Geometry check sheet. Reference: drawing and pictorial views, mm from the part's lowest x, y, z. Give positions to 0.01 mm unless a question says otherwise; leave off trailing zeros. Order: outer loops, then holes, each group sorted by start corner. A loop starts at its lowest first (then second) coordinate and runs counter-clockwise, first axis right, second up. Notation, with made-up numbers: (13, -25.75) -> (20, -25.75) arc R26 cw to (20, -7.75) -> close; hole circle Ø9 at (45, -3.5). An arc over 180 degrees is marked (long way). Write each question's results on one line, items separated by ' | '. Start each with the question number.
1. Cross-section at A-A, the plane x = 59. Enter the section's corners in (y, z).
2. Depth check by flat-ended pin: pin 1 Ø1 at (x, z) = (38.5, 1) entering from -Y. Enter the tip coordinate at first touch or a pass-through.
3. Cross-section at C-C, the plane y = 73. Enter the section's corners in (x, z), then the cut area to 3 significant figures.
4. Cross-section at D-D, the plane z = 0.55. State how many separate pieces and enclosed holes the cut face has, then the cut area to 3 significant figures.
5. Cross-section at B-B, the plane x = 12. Enter the section's corners in (y, z).
6. Material ranges on L1, parallel to Y at x = 12, z = 1.1; L2, parallel to Y at x = 43, z = 0.95; L3, parallel to Y at x = 59, z = 1.3, recorded low to high. Write a range as from..to.
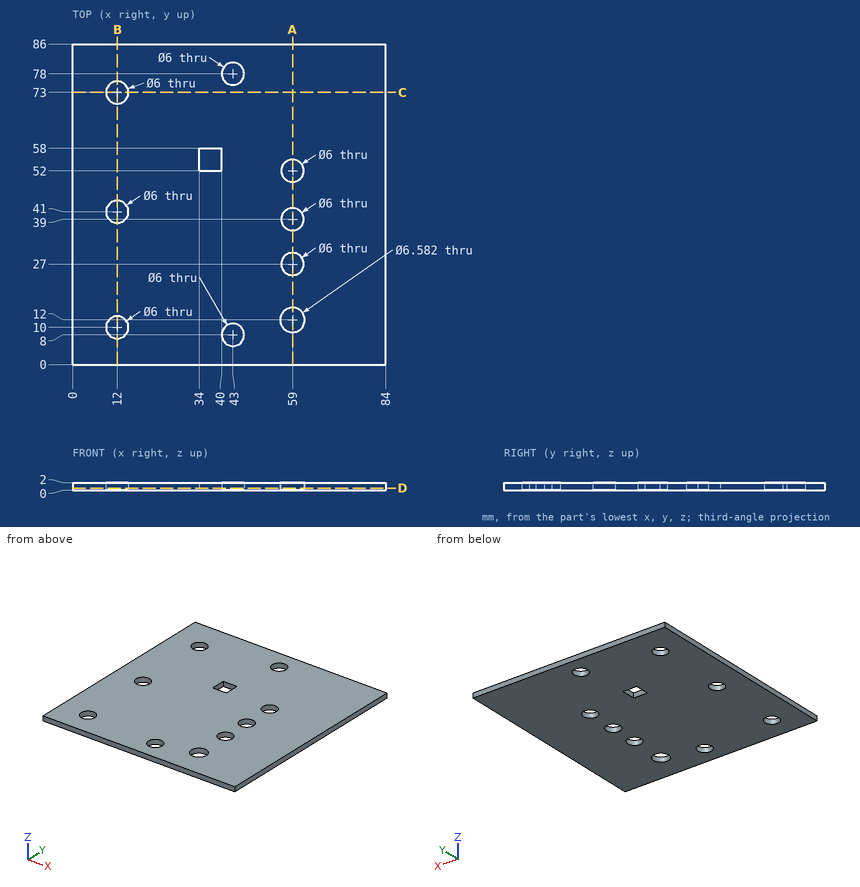
Results below:
1) outline: (0, 0) -> (8.71, 0) -> (8.71, 2) -> (0, 2) -> close; (15.29, 0) -> (24, 0) -> (24, 2) -> (15.29, 2) -> close; (30, 0) -> (36, 0) -> (36, 2) -> (30, 2) -> close; (42, 0) -> (49, 0) -> (49, 2) -> (42, 2) -> close; (55, 0) -> (86, 0) -> (86, 2) -> (55, 2) -> close
2) pin 1: stops at y = 0
3) outline: (0, 0) -> (9, 0) -> (9, 2) -> (0, 2) -> close; (15, 0) -> (84, 0) -> (84, 2) -> (15, 2) -> close | area: 156 mm²
4) separate pieces: 1 | enclosed holes: 10 | area: 6,930 mm²
5) outline: (0, 0) -> (7, 0) -> (7, 2) -> (0, 2) -> close; (13, 0) -> (38, 0) -> (38, 2) -> (13, 2) -> close; (44, 0) -> (70, 0) -> (70, 2) -> (44, 2) -> close; (76, 0) -> (86, 0) -> (86, 2) -> (76, 2) -> close
6) L1: y = 0..7, 13..38, 44..70, 76..86 | L2: y = 0..5, 11..75, 81..86 | L3: y = 0..8.71, 15.29..24, 30..36, 42..49, 55..86
